Autodesk Fusion 360 part; units mm, degrees
sketch "Sketch1" plane through (0, 0, 0) normal (0, 1, 0) x (1, 0, 0)
  line L0 (30, 30) -> (-30, 30)
  line L1 (-30, 30) -> (-30, -30)
  line L2 (-30, -30) -> (30, -30)
  line L3 (30, -30) -> (30, 30)
  line L4 (30, 30) -> (-30, -30) construction
  line L5 (-30, 30) -> (30, -30) construction
  dimension "d1" = 60
  dimension "d2" = 60
extrude "Extrude1" add sketch "Sketch1" along normal blind 12
chamfer "Chamfer1" distance 8 angle 45 1 edges at (30, 6, 30)
chamfer "Chamfer2" distance 8 angle 45 1 edges at (30, 6, -30)
chamfer "Chamfer3" distance 8 angle 45 1 edges at (-30, 6, 30)
chamfer "Chamfer4" distance 8 angle 45 1 edges at (-30, 6, -30)
Here's how the part is built. I have some questions about the finished solid (model axes, mm). Coordinates: 2 decimals unless noted, no trailing zeros. Loops run counter-clockwise (first coordinate to the right, second up) from the corner with the lowest first, then second, coordinate; pieces in that order, holes last. Notation, with made-up numbers: (41.25, 22) - (88.25, 22) arc R8 ccw to (88.25, 31) - close; hole circle Ø7 at (-38.5, 89.25). An arc over 180 degrees is marked (long way). Return JSON: item names as keys, results as strings. Group by question number.
Item 1: If we section it at B-B on x = 24.5: Write out the boundary of the cut face in (y, z).
Item 2: If we section it at C-C on z = -23: Write out the boundary of the cut face in (x, y).
Item 3: If we section it at A-A on y = 10: Write out the boundary of the cut face in (x, z), and give its area (3 significant figures).
Item 4: I need wall thicknesses on line 1 (X direction, y = 2, z = 25.5); line 2 (Z direction, x = -23, y = 2.25); line 3 (X direction, y = 4, z = 22.5). Which ranges of each line are inside material? Lowest first, please. Write a range as from..to.
Calculated:
{
 "1": {"outline": "(0, -27.5) - (12, -27.5) - (12, 27.5) - (0, 27.5) - close"},
 "2": {"outline": "(-29, 0) - (29, 0) - (29, 12) - (-29, 12) - close"},
 "3": {"outline": "(-30, -22) - (-22, -30) - (22, -30) - (30, -22) - (30, 22) - (22, 30) - (-22, 30) - (-30, 22) - close", "area": "3,470 mm^2"},
 "4": {"line 1": "x = -26.5..26.5", "line 2": "z = -29..29", "line 3": "x = -29.5..29.5"}
}
